Can you work these out from the model? Positions are in its coordinate system, mm. Give positions to 0.01 mm unless a question says otherwise; leave off trailing zeros. Order: outer loops, then holes, each group sorted by start corner. A loop starts at its lowest first (then second) coordinate and runs counter-clockwise, first axis right, second up. Notation, with made-up numbers: (25, 24.25) - (54, 24.25) arc R12 cw to (54, 46.25) - close; hole circle Ø8 at (54.25, 38). An arc over 180 degrees is marked (long way). Return JSON: item names as keys, results as strings.
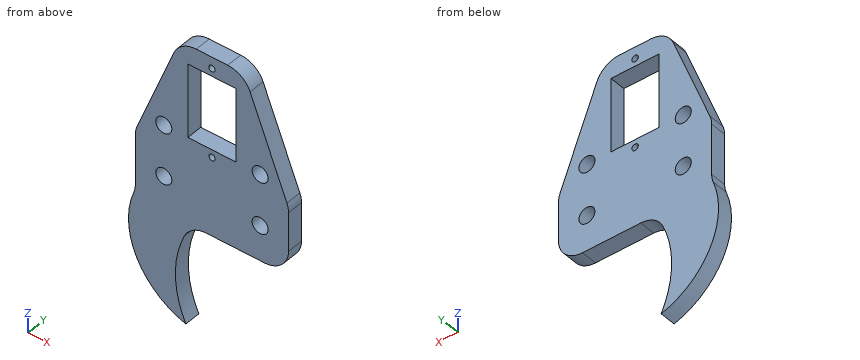
```python
from build123d import *

# Parameters (mm, degrees)
SKETCH1_R           = 25
BOSS_EXTRUDE1_DEPTH = 5
CUT_EXTRUDE1_DEPTH  = 5
BOSS_EXTRUDE2_DEPTH = 5
SKETCH7_W           = 20
SKETCH7_H           = 35
SKETCH7_R           = 1
SKETCH7_W_2         = 15
SKETCH7_H_2         = 23
BOSS_EXTRUDE3_DEPTH = 5
BOSS_EXTRUDE4_DEPTH = 5
SKETCH10_R          = 2.5
CUT_EXTRUDE3_DEPTH  = 5
FILLET3_R           = 7.5


with BuildPart() as part:
    # Sketch1 → Boss-Extrude1 (new body)
    with BuildSketch(Plane(origin=(0, 0, 0), x_dir=(1, 0, 0), z_dir=(0, 1, 0))):
        with Locations(Location((0, 0, 0), (0, 0, 270))):
            Circle(SKETCH1_R)
    extrude(amount=BOSS_EXTRUDE1_DEPTH)

    # Sketch2 → Cut-Extrude1 (cut)
    with BuildSketch(Plane(origin=(0, 5, 0), x_dir=(1, 0, 0), z_dir=(0, 1, 0))):
        with BuildLine():
            Line((49.553686115, 140.810270452), (-7.133634365, 23.960618956))
            ThreePointArc((-7.133634365, 23.960618956), (-7.596668184, -3.37247162), (12.986967165, -21.362085195))
            Line((12.986967165, -21.362085195), (137.676563898, -57.691106988))
            Line((137.676563898, -57.691106988), (375.081896712, 47.702827292))
            Line((375.081896712, 47.702827292), (286.959018929, 246.204204732))
            Line((286.959018929, 246.204204732), (49.553686115, 140.810270452))
        make_face()
    extrude(amount=-CUT_EXTRUDE1_DEPTH, mode=Mode.SUBTRACT)

    # Sketch4 → Boss-Extrude2 (add)
    with BuildSketch(Plane(origin=(0, 5, 0), x_dir=(1, 0, 0), z_dir=(0, 1, 0))):
        with BuildLine():
            Line((24.840469341, -7.763428106), (-5.227737426, -7.763428106))
            ThreePointArc((-5.227737426, -7.763428106), (2.650074831, -16.20966255), (12.986967165, -21.362085195))
            ThreePointArc((12.986967165, -21.362085195), (-7.468591232, -23.858334917), (-22.849556978, -10.143852617))
            Line((-22.849556978, -10.143852617), (-22.849556978, -28.782420825))
            Line((-22.849556978, -28.782420825), (24.840469341, -28.782420825))
            Line((24.840469341, -28.782420825), (24.840469341, -7.763428106))
        make_face()
    extrude(amount=-BOSS_EXTRUDE2_DEPTH)

    # Sketch7 → Boss-Extrude3 (add)
    with BuildSketch(Plane(origin=(0, 5, 0), x_dir=(1, 0, 0), z_dir=(0, 1, 0))):
        with Locations((0.995456182, -46.282420825)):
            Rectangle(SKETCH7_W, SKETCH7_H)
        with Locations(Location((0.995456182, -60.182420825, 0), (0, 0, 270))):
            Circle(SKETCH7_R, mode=Mode.SUBTRACT)
        with Locations(Location((0.995456182, -32.382420825, 0), (0, 0, 90))):
            Circle(SKETCH7_R, mode=Mode.SUBTRACT)
        with Locations((0.995456182, -46.282420825)):
            Rectangle(SKETCH7_W_2, SKETCH7_H_2, mode=Mode.SUBTRACT)
    extrude(amount=-BOSS_EXTRUDE3_DEPTH)

    # Sketch9 → Boss-Extrude4 (add)
    with BuildSketch(Plane(origin=(0, 5, 0), x_dir=(1, 0, 0), z_dir=(0, 1, 0))):
        Polygon((-22.849556978, -28.782420825), (-9.004543818, -63.782420825), (-9.004543818, -28.782420825), align=None)
        Polygon((10.995456182, -63.782420825), (24.840469341, -28.782420825), (10.995456182, -28.782420825), align=None)
    extrude(amount=-BOSS_EXTRUDE4_DEPTH)

    # Sketch10 → Cut-Extrude3 (cut)
    with BuildSketch(Plane(origin=(0, 5, 0), x_dir=(1, 0, 0), z_dir=(0, 1, 0))):
        with Locations(Location((15.995456182, -34.782420825, 0), (0, 0, 270))):
            Circle(SKETCH10_R)
        with Locations(Location((-14.004543818, -34.782420825, 0), (0, 0, 90))):
            Circle(SKETCH10_R)
        with Locations(Location((15.995456182, -18.782420825, 0), (0, 0, 90))):
            Circle(SKETCH10_R)
        with Locations(Location((-14.004543818, -18.782420825, 0), (0, 0, 270))):
            Circle(SKETCH10_R)
    extrude(amount=-CUT_EXTRUDE3_DEPTH, mode=Mode.SUBTRACT)

    # Fillet3
    fillet3_edges = [part.edges().sort_by_distance(p)[0] for p in [
        (-22.849556978, 2.5, 28.782420825),
        (-22.849556978, 2.5, 10.143852617),
        (-5.227737426, 2.5, 7.763428106),
        (24.840469341, 2.5, 7.763428106),
        (24.840469341, 2.5, 28.782420825),
        (10.995456182, 2.5, 63.782420825),
        (-9.004543818, 2.5, 63.782420825),
    ]]
    fillet(fillet3_edges, radius=FILLET3_R)


solid = part.part
```
1. Suppose I cut it at A-A (x = 3). List the corners of the cut face in (y, z) for me.
Checks:
{"outline": "(0, 7.76) - (5, 7.76) - (5, 34.78) - (0, 34.78) - close; (0, 57.78) - (5, 57.78) - (5, 63.78) - (0, 63.78) - close"}
2. For pin 1 Ø2 at (y, z) = (0.5, -1.5) entering from -X (3 decimals); pin 2 Ø2.5 at (x, y) = (4.5, 3.5) entering from -Z; pin 3 Ø1 at (y, z) = (3.5, 26.5) entering from -X, each with a flat end and sliding along its axis, tell me the tip position at first contact or that it passes through.
Checks:
{"pin 1": "x = -24.995", "pin 2": "z = 7.76", "pin 3": "x = -22.85"}
3. If I drill on L1, parallel to X at y = 3.95, z = 19; L2, parallel to Z at x = 3, y = 1.1; L3, parallel to X at y = 2.6, z = 20, over which ranges is the centre line in solid material (lowest first)? Write a range as [from, to].
Checks:
{"L1": "[-22.85, -16.5], [-11.51, 13.5], [18.49, 24.84]", "L2": "[7.76, 34.78], [57.78, 63.78]", "L3": "[-22.85, -16.19], [-11.82, 13.81], [18.18, 24.84]"}
4. Suppose I cut it at C-C (z = 17.5). List the corners of the cut face in (x, y) for me.
Checks:
{"outline": "(-22.85, 0) - (-16.15, 0) - (-16.15, 5) - (-22.85, 5) - close; (-11.86, 0) - (13.85, 0) - (13.85, 5) - (-11.86, 5) - close; (18.14, 0) - (24.84, 0) - (24.84, 5) - (18.14, 5) - close"}
5. Suppose I cut it at D-D (z = 53.5). List the corners of the cut face in (x, y) for me.
Checks:
{"outline": "(-13.07, 0) - (-6.5, 0) - (-6.5, 5) - (-13.07, 5) - close; (8.5, 0) - (15.06, 0) - (15.06, 5) - (8.5, 5) - close"}
6. Suppose I cut it at B-B (y = 1.5). List the corners of the cut face in (x, z) for me, plus the area to 3 significant figures.
Checks:
{"outline": "(-23.35, 8.94) arc R25 ccw to (-7.13, -23.96) arc R32.45 cw to (-7.63, 3.29) arc R7.5 cw to (-0.77, 7.76) - (17.34, 7.76) arc R7.5 ccw to (24.84, 15.26) - (24.84, 27.35) arc R7.5 ccw to (24.31, 30.11) - (12.87, 59.04) arc R7.5 ccw to (5.9, 63.78) - (-3.91, 63.78) arc R7.5 ccw to (-10.88, 59.04) - (-22.32, 30.11) arc R7.5 ccw to (-22.85, 27.35) - (-22.85, 11.63) arc R7.5 cw to start; hole circle Ø5 at (-14, 18.78); hole circle Ø5 at (-14, 34.78); hole (-6.5, 34.78) - (8.5, 34.78) - (8.5, 57.78) - (-6.5, 57.78) - close; hole circle Ø2 at (1, 32.38); hole circle Ø2 at (1, 60.18); hole circle Ø5 at (16, 18.78); hole circle Ø5 at (16, 34.78)", "area": "2,130 mm^2"}
